For this review, take the finished solid that the model builds, in its own axes (mm). Give positions to 0.01 mm unless a question says otherwise; leave off trailing zeros. Order: outer loops, then holes, each group sorted by start corner. A loop starts at its lowest first (then second) coordinate and runs counter-clockwise, first axis right, second up. Notation, with made-up numbers: (54.5, -26) - (98.5, -26) arc R12 cw to (98.5, -22) - close; hole circle Ø5 at (31.5, 50). An arc over 180 degrees is marked (long way). Use a Markdown table: item, result. Add a question column.
1) Wall thickness on L1, parallel to Y at x = 1.5, z = 73.5; L2, parallel to Y at x = -13.5, z = 79.5: over which ranges is each line inside the solid? List them lowest first.
2) We need section A-A on y = 18.5. Give the number of separate pieces and of enclosed holes in the cut face, then the cut area to 3 significant figures.
3) We need section B-B on x = 18. Write out the cut boundary in (y, z), then the cut area to 3 significant figures.
4) Clearance check with flat-ended pins moving along their axes: P1, Ø5.5, axis at x = 9, z = 112.5, coming from the +Y side; P2, Ø5, axis at x = 0.5, z = 86.5, coming from the +Y side. State where each tip first meets the part, or that it passes through.
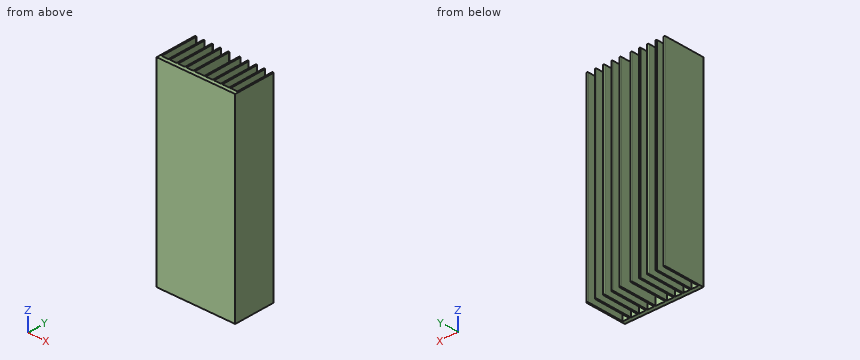
```python
from build123d import *

# Parameters (mm, degrees)
SALIENTE_EXTRUIR1_DEPTH = 200
MATRIZL1_COUNT          = 5
MATRIZL1_PITCH          = 8.4
SIMETR_A1_COPY_1_DEPTH  = 200
SIMETR_A1_COPY_2_DEPTH  = 200
SIMETR_A1_COPY_3_DEPTH  = 200
SIMETR_A1_COPY_4_DEPTH  = 200


with BuildPart() as part:
    # Croquis1 → Saliente-Extruir1 (new body)
    with BuildSketch(Plane.XY):
        with BuildLine():
            Line((31.6, 4), (31.6, 0))
            Line((31.6, 0), (40, 0))
            Line((40, 0), (40, 42))
            ThreePointArc((40, 42), (39.25, 42.75), (38.5, 42))
            Line((38.5, 42), (38.5, 4))
            Line((38.5, 4), (31.6, 4))
        make_face()
    saliente_extruir1 = extrude(amount=SALIENTE_EXTRUIR1_DEPTH)

    # MatrizL1: Saliente-Extruir1 ×5
    with Locations(*[(-i * MATRIZL1_PITCH, 0, 0) for i in range(1, MATRIZL1_COUNT)]):
        add(saliente_extruir1)



with BuildPart() as simetr_a1_1:
    # Simetr_a1: Saliente-Extruir1 across plane
    add(saliente_extruir1.mirror(Plane(origin=(0, 0, 0), x_dir=(0, 0, 1), z_dir=(1, 0, 0))))

    # Simetr_a1 copy 1 sketch → Simetr_a1 copy 1 (add)
    with BuildSketch(Plane(origin=(8.4, 0, 0), x_dir=(-1, 0, 0), z_dir=(0, 0, 1))):
        with BuildLine():
            Line((31.6, -4), (31.6, 0))
            Line((31.6, 0), (40, 0))
            Line((40, 0), (40, -42))
            ThreePointArc((40, -42), (39.25, -42.75), (38.5, -42))
            Line((38.5, -42), (38.5, -4))
            Line((38.5, -4), (31.6, -4))
        make_face()
    extrude(amount=SIMETR_A1_COPY_1_DEPTH)

    # Simetr_a1 copy 2 sketch → Simetr_a1 copy 2 (add)
    with BuildSketch(Plane(origin=(16.8, 0, 0), x_dir=(-1, 0, 0), z_dir=(0, 0, 1))):
        with BuildLine():
            Line((31.6, -4), (31.6, 0))
            Line((31.6, 0), (40, 0))
            Line((40, 0), (40, -42))
            ThreePointArc((40, -42), (39.25, -42.75), (38.5, -42))
            Line((38.5, -42), (38.5, -4))
            Line((38.5, -4), (31.6, -4))
        make_face()
    extrude(amount=SIMETR_A1_COPY_2_DEPTH)

    # Simetr_a1 copy 3 sketch → Simetr_a1 copy 3 (add)
    with BuildSketch(Plane(origin=(25.2, 0, 0), x_dir=(-1, 0, 0), z_dir=(0, 0, 1))):
        with BuildLine():
            Line((31.6, -4), (31.6, 0))
            Line((31.6, 0), (40, 0))
            Line((40, 0), (40, -42))
            ThreePointArc((40, -42), (39.25, -42.75), (38.5, -42))
            Line((38.5, -42), (38.5, -4))
            Line((38.5, -4), (31.6, -4))
        make_face()
    extrude(amount=SIMETR_A1_COPY_3_DEPTH)


with BuildPart() as part_1:
    add(part.part)

    add(simetr_a1_1.part)  # Simetr_a1 copy 4 merges Simetr_a1_1
    # Simetr_a1 copy 4 sketch → Simetr_a1 copy 4 (add)
    with BuildSketch(Plane(origin=(33.6, 0, 0), x_dir=(-1, 0, 0), z_dir=(0, 0, 1))):
        with BuildLine():
            Line((31.6, -4), (31.6, 0))
            Line((31.6, 0), (40, 0))
            Line((40, 0), (40, -42))
            ThreePointArc((40, -42), (39.25, -42.75), (38.5, -42))
            Line((38.5, -42), (38.5, -4))
            Line((38.5, -4), (31.6, -4))
        make_face()
    extrude(amount=SIMETR_A1_COPY_4_DEPTH)


solid = part_1.part
```
Checked values:
| question | item | result |
|---|---|---|
| 1 | L1 | 0 to 4 |
| 1 | L2 | 0 to 42.51 |
| 2 | separate pieces | 10 |
| 2 | enclosed holes | 0 |
| 2 | area | 3,000 mm² |
| 3 | outline | (0, 0) - (4, 0) - (4, 200) - (0, 200) - close |
| 3 | area | 800 mm² |
| 4 | P1 | y = 42.45 |
| 4 | P2 | y = 4 |
